Geometry check sheet. Reference: the model listing, model coordinates, mm. Face numbers are marked on the shaded views. A direction names the side the tool comes from. Round coordinates to 2 decimals unless told otherwise and drop trailing zeros. Order: outer loops, then holes, each group sorted by start corner. A loop starts at its lowest first (then second) coordinate and runs counter-clockwise, first axis right, second up. Notation, with made-up numbers: (30, 36.5) - (44, 36.5) arc R25 cw to (44, 71.5) - close; hole circle Ø7 at (76, -16.75). An arc over 180 degrees is marked (long way). Write each question's results on one line, items separated by ' | '.
```python
from build123d import *

# Parameters (mm, degrees)
F1_DEPTH = 25.4
F2_R     = 3.81
F2_R_2   = 5.08
F2_R_3   = 6.35
F3_DEPTH = 71.1383146132


# Not quite as in the source:
# - a feature names something its author has since deleted; it is built from what else it names


with BuildPart() as f1:
    # F0 (on Front) → F1 (new body)
    with BuildSketch(Plane.XZ):
        with BuildLine():
            Line((-5.08, 0), (0, 0))
            Line((0, 0), (0, 38.1))
            Line((0, 38.1), (0, 40.6573146132))
            ThreePointArc((0, 40.6573146132), (7.4394877579, 58.6178268553), (25.4, 66.0573146132))
            Line((25.4, 66.0573146132), (86.36, 66.0573146132))
            Line((86.36, 66.0573146132), (86.36, 71.1373146132))
            Line((86.36, 71.1373146132), (0, 71.1373146132))
            Line((0, 71.1373146132), (-2.54, 71.1373146132))
            ThreePointArc((-2.54, 71.1373146132), (-16.9084097937, 65.1857244069), (-22.86, 50.8173146132))
            Line((-22.86, 50.8173146132), (-22.86, 43.18))
            Line((-22.86, 43.18), (-5.08, 60.96))
            Line((-5.08, 60.96), (-5.08, 0))
        make_face()
    extrude(amount=F1_DEPTH)

    # F2 (on face) → F3 (cut, through all)
    with BuildSketch(Plane.XY.offset(71.1373146132)):
        with Locations((77.47, -12.7)):
            Circle(F2_R)
        with Locations((46.99, -12.7)):
            Circle(F2_R_2)
        with Locations((12.7, -12.7)):
            Circle(F2_R_3)
    extrude(amount=-F3_DEPTH, mode=Mode.SUBTRACT)


solid = f1.part
```
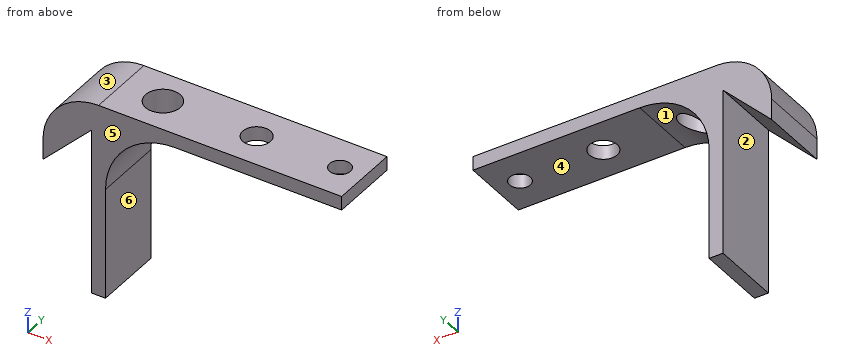
(1) Draft check along X on the marked faces 1, 2, 3 and 4. Enter one of: released by +X, released by -X, zero draft, split by the parting line, or undercut.
Answers follow:
face 1: released by +X | face 2: undercut | face 3: released by -X | face 4: zero draft
(2) Access from +Z, -Z, +X, -X, +Y, -Y to the whole of each face (thin tool, end or side, straight path). Record for the marked faces 5 and 6.
Answers follow:
face 5: +Z, -Z, +X, -X, -Y | face 6: -Z, +X, +Y, -Y
(3) Section check B-B (y = -10). Record the cut outline in (x, z).
Answers follow:
outline: (-22.86, 43.18) - (-5.08, 60.96) - (-5.08, 0) - (0, 0) - (0, 40.66) arc R25.4 cw to (6.95, 58.12) - (6.95, 71.14) - (-2.54, 71.14) arc R20.32 ccw to (-22.86, 50.82) - close; (18.45, 65.09) arc R25.4 cw to (25.4, 66.06) - (42.69, 66.06) - (42.69, 71.14) - (18.45, 71.14) - close; (51.29, 66.06) - (74.78, 66.06) - (74.78, 71.14) - (51.29, 71.14) - close; (80.16, 66.06) - (86.36, 66.06) - (86.36, 71.14) - (80.16, 71.14) - close
(4) Material ranges on line 1 (Y direction, x = 77.47, z = 69); line 2 (Y direction, x = 46.99, z = 69.2); line 3 (X direction, y = -10.25, z = 17), recorded low to high.
Answers follow:
line 1: -25.4 to -16.51, -8.89 to 0 | line 2: -25.4 to -17.78, -7.62 to 0 | line 3: -5.08 to 0
(5) Section check A-A (x = 77.47). Record the cut outline in (y, z).
Answers follow:
outline: (-25.4, 66.06) - (-16.51, 66.06) - (-16.51, 71.14) - (-25.4, 71.14) - close; (-8.89, 66.06) - (0, 66.06) - (0, 71.14) - (-8.89, 71.14) - close
(6) Section check D-D (y = -2). Record the cut outline in (x, z).
Answers follow:
outline: (-22.86, 43.18) - (-5.08, 60.96) - (-5.08, 0) - (0, 0) - (0, 40.66) arc R25.4 cw to (25.4, 66.06) - (86.36, 66.06) - (86.36, 71.14) - (-2.54, 71.14) arc R20.32 ccw to (-22.86, 50.82) - close
(7) Depth check by flat-ended pin: pin 1 Ø7.5 at (y, z) = (-18.5, 26.5) entering from +X; pin 2 Ø6 at (x, y) = (55, -13.5) entering from -Z. Enter the tip coordinate at first touch or a pass-through.
Answers follow:
pin 1: x = 0 | pin 2: z = 66.06
(8) Section check C-C (z = 44.5). Record the cut outline in (x, y).
Answers follow:
outline: (-22.86, -25.4) - (-21.54, -25.4) - (-21.54, 0) - (-22.86, 0) - close; (-5.08, -25.4) - (0.29, -25.4) - (0.29, 0) - (-5.08, 0) - close
